Model file for the job. Use its own axes, mm. Round coordinates to 2 decimals unless told otherwise and drop trailing zeros. Order: outer loops, then holes, each group sorted by start corner. A loop starts at its lowest first (then second) coordinate and runs counter-clockwise, first axis right, second up. Notation, with made-up numbers: M 72.5,-18.75 L 125.5,-18.75 A13 cw 125.5,0.25 Z; hole C 54.25,39.5 d10. An arc over 180 degrees is marked long. Return JSON: item names as keys, results as strings. Group by question number.
Item 1: Pin check, flat tips, straight feed: pin 1 Ø2 at (y, z) = (1.5, 20.5) entering from -X; pin 2 Ø1.8 at (x, z) = (0, -12.5) entering from +Y; pin 3 Ø3 at (y, z) = (2, 4.5) entering from -X. Stop position of each tip, or through.
Item 2: Slice it at A-A on z = 0. Write the cut outline in (x, y).
Item 3: Slice it at B-B on y = 3.2. Give the number of separate pieces and of enclosed holes in the cut face, then the cut area to 3 significant figures.
Item 4: Pull direction Z, two halves, no side cores. Call faces 1 (the face through (36, 5, -1)), 2 (the face through (156.93, 2.46, 2.87)), 3 (the face through (158.642, 2.465, 9.031)): pulls with the +Z half, pulls with the -Z half, needs draft (parallel to the pull), parting line crosses it, or undercut.
Item 5: Probe line 1 along X through (y, z) = (2, 28.5); line 2 along Z through (x, y) = (0.5, 2); line 3 along X through (y, z) = (3.7, -6.25). List the from-to ranges inside material, lowest first.
from build123d import *

# Parameters (mm, degrees)
BOSS_EXTRUDE3_OUTLINE_R = 7.5
BOSS_EXTRUDE3_DEPTH     = 5
SKETCH2_R               = 1.5
CUT_EXTRUDE1_DEPTH      = 10
SKETCH3_R               = 1.5
CUT_EXTRUDE2_DEPTH      = 10
SKETCH4_R               = 1.5
CUT_EXTRUDE3_DEPTH      = 10


# Read off the part's stored shape, not the designer's step: Boss-Extrude3
with BuildPart() as part:
    # Boss-Extrude3 outline → Boss-Extrude3 (new body)
    with BuildSketch(Plane(origin=(0, 0, 0), x_dir=(1, 0, 0), z_dir=(0, 1, 0))):
        with BuildLine():
            ThreePointArc((0, 42.5), (-42.5, 0), (0, -42.5))
            add(Edge.make_bspline(
                [(0, -42.5), (35.287909835, -42.5), (94.296573589, 3.71849472), (141.161165235, -8.838834765)],
                knots=[0, 0, 0, 0, 1, 1, 1, 1], degree=3))
            ThreePointArc((141.161165235, -8.838834765), (158.838834765, -8.838834765), (158.838834765, 8.838834765))
            add(Edge.make_bspline(
                [(0, 42.5), (43.860357416, 42.5), (128.226009794, 39.451659736), (158.838834765, 8.838834765)],
                knots=[0, 0, 0, 0, 1, 1, 1, 1], degree=3))
        make_face()
        with Locations((150, 0)):
            Circle(BOSS_EXTRUDE3_OUTLINE_R, mode=Mode.SUBTRACT)
    extrude(amount=BOSS_EXTRUDE3_DEPTH)

    # Sketch2 → Cut-Extrude1 (cut)
    with BuildSketch(Plane(origin=(0, 5, 0), x_dir=(1, 0, 0), z_dir=(0, 1, 0))):
        with Locations(Location((0, 35, 0), (0, 0, 270))):
            Circle(SKETCH2_R)
        with Locations(Location((0, 12.5, 0), (0, 0, 270))):
            Circle(SKETCH2_R)
        with Locations(Location((10.825317547, 6.25, 0), (0, 0, 270))):
            Circle(SKETCH2_R)
        with Locations(Location((10.825317547, -6.25, 0), (0, 0, 270))):
            Circle(SKETCH2_R)
        with Locations(Location((0, -12.5, 0), (0, 0, 270))):
            Circle(SKETCH2_R)
        with Locations(Location((-10.825317547, -6.25, 0), (0, 0, 270))):
            Circle(SKETCH2_R)
        with Locations(Location((-10.825317547, 6.25, 0), (0, 0, 270))):
            Circle(SKETCH2_R)
        with Locations(Location((-20.57248383, 28.315594803, 0), (0, 0, 270))):
            Circle(SKETCH2_R)
        with Locations(Location((-33.28697807, 10.815594803, 0), (0, 0, 270))):
            Circle(SKETCH2_R)
        with Locations(Location((-33.28697807, -10.815594803, 0), (0, 0, 270))):
            Circle(SKETCH2_R)
        with Locations(Location((-20.57248383, -28.315594803, 0), (0, 0, 270))):
            Circle(SKETCH2_R)
        with Locations(Location((0, -35, 0), (0, 0, 270))):
            Circle(SKETCH2_R)
    extrude(amount=-CUT_EXTRUDE1_DEPTH, mode=Mode.SUBTRACT)

    # Sketch3 → Cut-Extrude2 (cut)
    with BuildSketch(Plane(origin=(0, 5, 0), x_dir=(1, 0, 0), z_dir=(0, 1, 0))):
        with Locations(Location((29.822508304, 35, 0), (0, 0, 270))):
            Circle(SKETCH3_R)
        with Locations(Location((57.312909887, 35, 0), (0, 0, 270))):
            Circle(SKETCH3_R)
    extrude(amount=-CUT_EXTRUDE2_DEPTH, mode=Mode.SUBTRACT)

    # Sketch4 → Cut-Extrude3 (cut)
    with BuildSketch(Plane(origin=(0, 5, 0), x_dir=(1, 0, 0), z_dir=(0, 1, 0))):
        with Locations(Location((35.461413578, -21.530349116, 0), (0, 0, 270))):
            Circle(SKETCH4_R)
        with Locations(Location((22.392043347, -28.36049342, 0), (0, 0, 270))):
            Circle(SKETCH4_R)
    extrude(amount=-CUT_EXTRUDE3_DEPTH, mode=Mode.SUBTRACT)


solid = part.part
Output values:
{
 "1": {"pin 1": "x = -37.76", "pin 2": "through", "pin 3": "x = -42.39"},
 "2": {"outline": "M -42.5,0 L 142.5,0 L 142.5,5 L -42.5,5 Z; M 157.5,0 L 162.5,0 L 162.5,5 L 157.5,5 Z"},
 "3": {"separate pieces": "1", "enclosed holes": "17", "area": "11,300 mm²"},
 "4": {"face 1": "needs draft", "face 2": "undercut", "face 3": "parting line crosses it"},
 "5": {"line 1": "-31.53 to -22.06, -19.08 to 20.9, 23.89 to 47.91", "line 2": "-42.5 to -36.41, -33.59 to -13.91, -11.09 to 11.09, 13.91 to 33.59, 36.41 to 42.5", "line 3": "-42.04 to -12.33, -9.33 to 9.33, 12.33 to 145.85, 154.15 to 160.83"}
}
